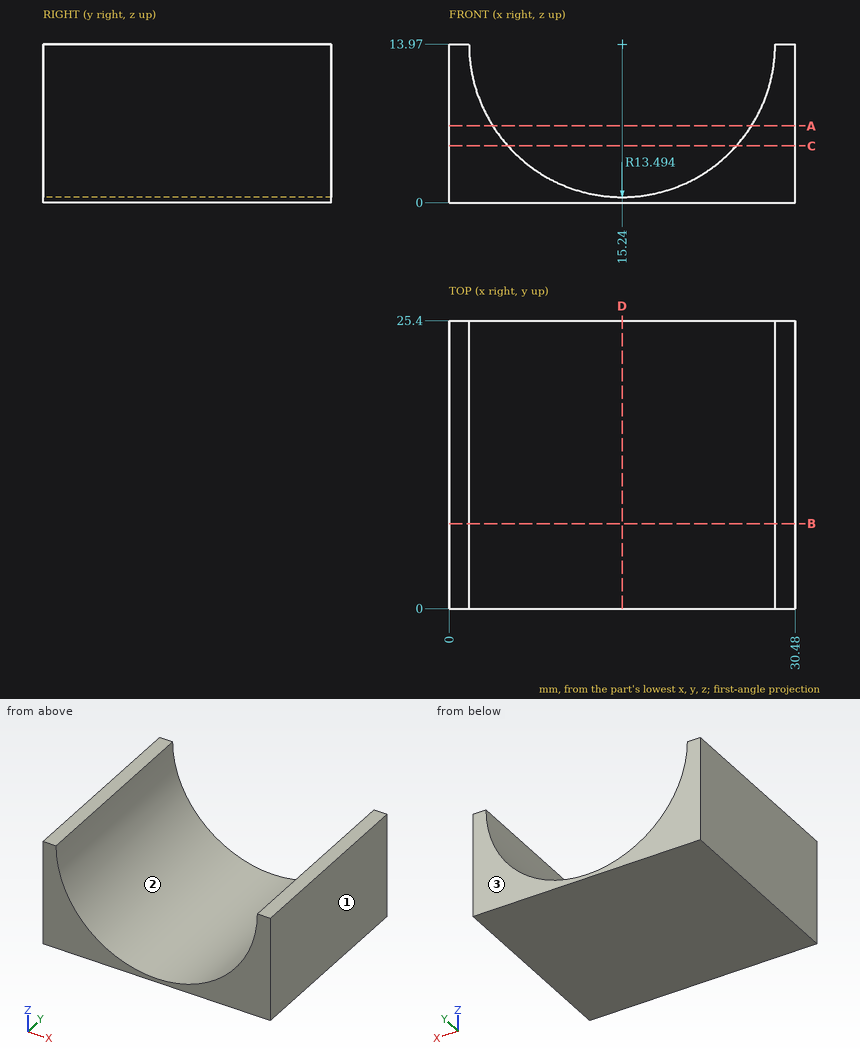
Answer from the drawing. Dimensions are ordinates in mm from the lowest x, y and z of the part. Give positions to 0.01 mm unless a question says otherwise; leave off trailing zeros. Loops run counter-clockwise (first coordinate to the right, second up) from the corner with the lowest first, then second, coordinate; pieces in that order, holes last. Notation, with made-up numbers: (63.25, 83.5) -> (116.25, 83.5) arc R28 cw to (116.25, 102.5) -> close; hole circle Ø2 at (14, -39.5). An arc over 180 degrees is marked (long way). Answer as CSV lines item,"result".
Item 1: This flat-tipped pin is pushed along its axis until it touches: pin 1 (10 mm diameter, centred on x = 9.5, y = 12, fed in from +Z). Where does it stop, or does it pass through?
Returned:
pin 1,"stops at z = 5.8"
Item 2: Find section C-C on z = 5. Give the vertices of the cut face in (x, y).
Returned:
outline,"(0, 0) -> (5.16, 0) -> (5.16, 25.4) -> (0, 25.4) -> close; (25.32, 0) -> (30.48, 0) -> (30.48, 25.4) -> (25.32, 25.4) -> close"
Item 3: Find section A-A on z = 6.75. Give the vertices of the cut face in (x, y), plus the area to 3 significant figures.
Returned:
outline,"(0, 0) -> (3.84, 0) -> (3.84, 25.4) -> (0, 25.4) -> close; (26.64, 0) -> (30.48, 0) -> (30.48, 25.4) -> (26.64, 25.4) -> close"
area,"195 mm²"
Item 4: Find section B-B on y = 7.5. Give the vertices of the cut face in (x, z).
Returned:
outline,"(0, 0) -> (30.48, 0) -> (30.48, 13.97) -> (28.73, 13.97) arc R13.49 cw to (1.75, 13.97) -> (0, 13.97) -> close"
Item 5: Determine the mould class of the marked faces 1, 2 and 3 for opening direction X: +X half, -X half, draft (parallel to the pull), parting line (faces both ways), or undercut.
Returned:
face 1,"+X half"
face 2,"undercut"
face 3,"draft"
Item 6: Find section D-D on x = 15.24. Give the vertices of the cut face in (y, z), plus the area to 3 significant figures.
Returned:
outline,"(0, 0) -> (25.4, 0) -> (25.4, 0.48) -> (0, 0.48) -> close"
area,"12.1 mm²"
Item 7: Consider line 1 (X direction, y = 17.25, z = 6.25); line 2 (X direction, y = 11.25, z = 10); line 3 (Z direction, x = 21.5, y = 12.5). Determine where each line is inside the solid, lowest interval first. Write a range as [from, to].
Returned:
line 1,"x = [0, 4.17], [26.31, 30.48]"
line 2,"x = [0, 2.34], [28.14, 30.48]"
line 3,"z = [0, 2.02]"
